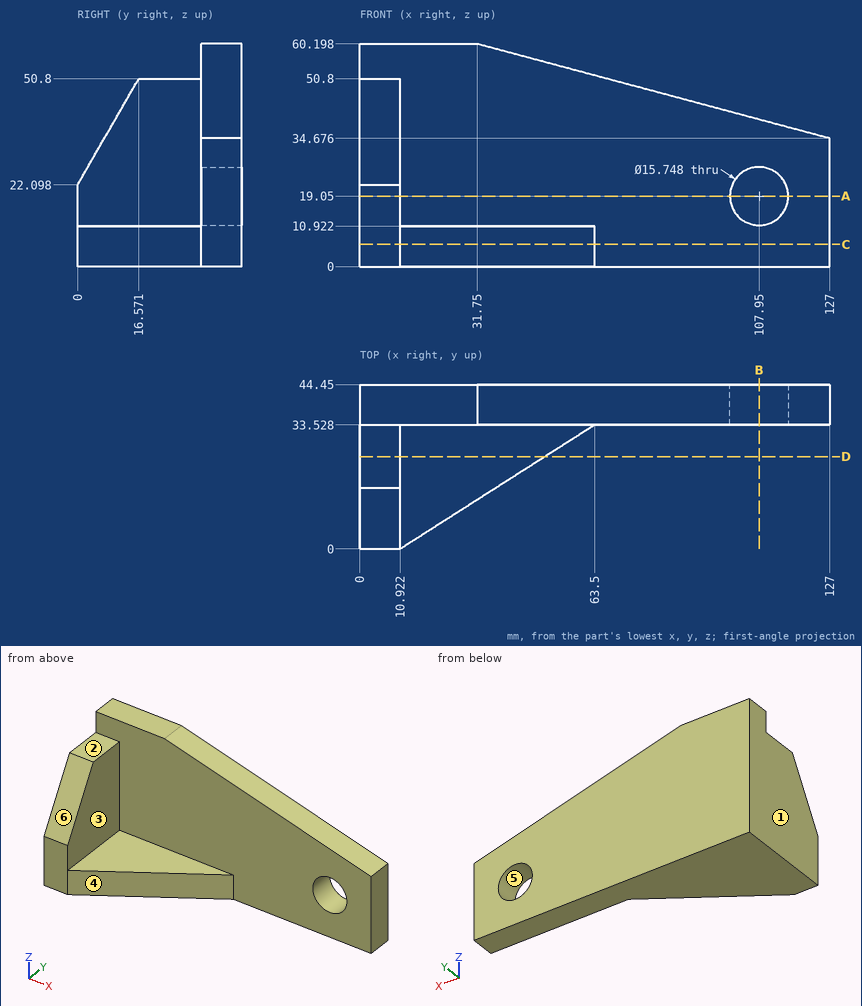
Answer from the drawing. Dimensions are ordinates in mm from the lowest x, y and z of the part. A direction names the side the tool comes from. Round coordinates to 2 decimals unless told otherwise and drop trailing zeros. Write each loop counter-clockwise with the first axis right and the second up, starting at its lowest first coordinate (ties: lowest second). Pieces come first, ordered by that corner, then holes. Notation, with made-up numbers: M 43.5,-35.75 L 86.5,-35.75 A21 ccw 86.5,-17.75 Z; hole C 89,-0.75 d2. An arc over 180 degrees is marked long. Write each question's results on one line, items separated by ' | '. Start each with the question number.
Item 1: Find section D-D on y = 25. Write down the section's boundary in (x, z), and give its area (3 significant figures).
Item 2: Find section A-A on z = 19.05. Write down the section's boundary in (x, y), and give its area (3 significant figures).
Item 3: Which of the six approach directions +Z, -Z, +X, -X, +Y, -Y give full straight-line access (tool end or side, diameter ignored) to the marked faces 1, 2 and 3?
Item 4: Find section B-B on x = 107.95. Write down the section's boundary in (y, z).
Item 5: The mould has two halves that part along X. Classify the marked faces 4, 5 and 6: +X half, -X half, draft (parallel to the pull), parting line (faces both ways), or undercut.
Item 6: Given pin 1 Ø12 at (x, z) = (22.5, 12.5) entering from -Y; pin 2 Ø5 at (x, z) = (77.5, 45) entering from -Y; pin 3 Ø9.5 at (x, z) = (107.95, 19.05) entering from -Y (1 decimal); pin 4 Ø3 at (y, z) = (17, 26) entering from +X, each flat-ended and moving along its own axis, determine where each tip first touches the part or whether it passes through.
Item 7: Straight lines are drawn through the part: probe 1 along X at (y, z) = (39, 19); probe 2 along Y at (x, z) = (37.5, 45); probe 3 along Z at (x, y) = (40.5, 23.5). For each, find the intervals that lie inside material, in ascending order.
Item 8: Find section C-C on z = 6. Write down the section's boundary in (x, y), and give its area (3 significant figures).
Answer block:
1) outline: M 0,0 L 50.13,0 L 50.13,10.92 L 10.92,10.92 L 10.92,50.8 L 0,50.8 Z | area: 983 mm²
2) outline: M 0,0 L 10.92,0 L 10.92,33.53 L 100.08,33.53 L 100.08,44.45 L 0,44.45 Z; M 115.82,33.53 L 127,33.53 L 127,44.45 L 115.82,44.45 Z | area: 1,580 mm²
3) face 1: +Z, -Z, -X, +Y, -Y | face 2: +Z, +X, -X, -Y | face 3: +Z, +X, -Y
4) outline: M 33.53,0 L 44.45,0 L 44.45,11.18 L 33.53,11.18 Z; M 33.53,26.92 L 44.45,26.92 L 44.45,39.78 L 33.53,39.78 Z
5) face 4: +X half | face 5: undercut | face 6: draft
6) pin 1: stops at y = 3.69 | pin 2: stops at y = 33.53 | pin 3: passes through | pin 4: stops at x = 10.92
7) probe 1: x = 0 to 100.08, 115.82 to 127 | probe 2: y = 33.53 to 44.45 | probe 3: z = 0 to 10.92
8) outline: M 0,0 L 10.92,0 L 63.5,33.53 L 127,33.53 L 127,44.45 L 0,44.45 Z | area: 2,630 mm²
